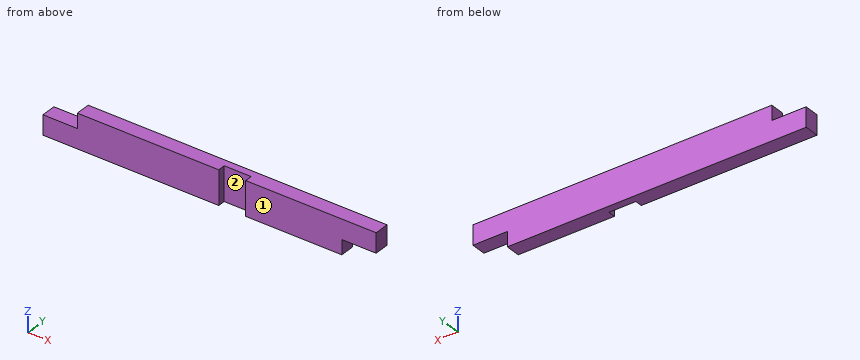
```python
from build123d import *

# Parameters (mm, degrees)
SKETCH1_W           = 863.6
SKETCH1_H           = 88.9
BOSS_EXTRUDE1_DEPTH = 38.1
SKETCH3_W           = 88.9
SKETCH3_H           = 38.1
CUT_EXTRUDE2_DEPTH  = 39.1
SKETCH4_W           = 69.85
SKETCH4_H           = 19.05
CUT_EXTRUDE3_DEPTH  = 89.9
SKETCH5_W           = 88.9
SKETCH5_H           = 38.1
CUT_EXTRUDE4_DEPTH  = 39.1


with BuildPart() as part:
    # Sketch1 → Boss-Extrude1 (new body)
    with BuildSketch(Plane(origin=(0, 0, 0), x_dir=(1, 0, 0), z_dir=(0, 1, 0))):
        with Locations((431.8, 44.45)):
            Rectangle(SKETCH1_W, SKETCH1_H)
    extrude(amount=BOSS_EXTRUDE1_DEPTH)

    # Sketch3 → Cut-Extrude2 (cut, through all)
    with BuildSketch(Plane(origin=(0, 38.1, 0), x_dir=(1, 0, 0), z_dir=(0, 1, 0))):
        with Locations((819.15, 69.85)):
            Rectangle(SKETCH3_W, SKETCH3_H)
    extrude(amount=-CUT_EXTRUDE2_DEPTH, mode=Mode.SUBTRACT)

    # Sketch4 → Cut-Extrude3 (cut, through all)
    with BuildSketch(Plane(origin=(0, 0, -88.9), x_dir=(-1, 0, 0), z_dir=(0, 0, -1))):
        with Locations((-490.5375, 9.525)):
            Rectangle(SKETCH4_W, SKETCH4_H)
    extrude(amount=-CUT_EXTRUDE3_DEPTH, mode=Mode.SUBTRACT)

    # Sketch5 → Cut-Extrude4 (cut, through all)
    with BuildSketch(Plane.XZ):
        with Locations((44.45, -19.05)):
            Rectangle(SKETCH5_W, SKETCH5_H)
    extrude(amount=-CUT_EXTRUDE4_DEPTH, mode=Mode.SUBTRACT)


solid = part.part
```
Check sheet for the modelled part. Datum: model origin and axes. Units: mm. Face numbers are marked on the shaded views. Give positions to 0.01 mm unless a question says otherwise; leave off trailing zeros. Loops run counter-clockwise (first coordinate to the right, second up) from the corner with the lowest first, then second, coordinate; pieces in that order, holes last. Notation, with made-up numbers: M 61,-36 L 111,-36 A21 cw 111,-21 Z; hole C -38.75,-15 d4. An arc over 180 degrees is marked long. Answer as CSV lines item,"result".
Item 1: Depth check by flat-ended pin: pin 1 Ø2 at (y, z) = (4.5, -9) entering from -X; pin 2 Ø19 at (y, z) = (13, -77) entering from +X; pin 3 Ø21 at (x, z) = (496.5, -22.5) entering from -Y. Enter the tip coordinate at first touch or a pass-through.
Reply:
pin 1,"x = 88.9"
pin 2,"x = 774.7"
pin 3,"y = 19.05"
Item 2: Sectioned sample at B-B, the plane z = -19. Enter the section's corners in (x, y), then the cut area to 3 significant figures.
Reply:
outline,"M 88.9,0 L 455.61,0 L 455.61,19.05 L 525.46,19.05 L 525.46,0 L 863.6,0 L 863.6,38.1 L 88.9,38.1 Z"
area,"28,200 mm^2"
Item 3: Scan lines: L1, parallel to X at y = 10.5, z = -75; L2, parallel to X at y = 14.5, z = -4; L3, parallel to X at y = 36.5, z = -84.5. Record each from-to range of solid material in increasing order.
Reply:
L1,"0 to 455.61, 525.46 to 774.7"
L2,"88.9 to 455.61, 525.46 to 863.6"
L3,"0 to 774.7"
Item 4: Sectioned sample at A-A, the plane y = 6. Enter the section's corners in (x, z), then the cut area to 3 significant figures.
Reply:
outline,"M 0,-88.9 L 455.61,-88.9 L 455.61,0 L 88.9,0 L 88.9,-38.1 L 0,-38.1 Z; M 525.46,-88.9 L 774.7,-88.9 L 774.7,-50.8 L 863.6,-50.8 L 863.6,0 L 525.46,0 Z"
area,"63,800 mm^2"
Item 5: Draft check along X on the marked faces 1 and 2. Enter one of: pulls with the +X half, pulls with the -X half, needs draft (parallel to the pull), parting line crosses it, or undercut.
Reply:
face 1,"needs draft"
face 2,"undercut"
Item 6: Sectioned sample at C-C, the plane x = 782. Enter the section's corners in (y, z).
Reply:
outline,"M 0,-50.8 L 38.1,-50.8 L 38.1,0 L 0,0 Z"
